from build123d import *

# Parameters (mm, degrees)
SKETCH1_W           = 12
SKETCH1_H           = 12
SKETCH1_W_2         = 3.175
SKETCH1_H_2         = 6
SKETCH1_W_3         = 6
SKETCH1_H_3         = 3.125
BOSS_EXTRUDE1_DEPTH = 1.5875


with BuildPart() as part:
    # Sketch1 → Boss-Extrude1 (new, symmetric)
    with BuildSketch(Plane.XY):
        Polygon((45.675, 0), (45.675, 4.5), (42.5, 4.5), (42.5, 13.5), (45.675, 13.5), (45.675, 22.5), (42.5, 22.5), (42.5, 31.5), (-42.5, 31.5), (-42.5, 22.5), (-45.675, 22.5), (-45.675, 13.5), (-42.5, 13.5), (-42.5, 4.5), (-45.675, 4.5), (-45.675, -4.5), (-42.5, -4.5), (-42.5, -13.5), (-45.675, -13.5), (-45.675, -22.5), (-42.5, -22.5), (-42.5, -31.5), (42.5, -31.5), (42.5, -22.5), (45.675, -22.5), (45.675, -13.5), (42.5, -13.5), (42.5, -4.5), (45.675, -4.5), align=None)
        with Locations((0, -16.5)):
            Rectangle(SKETCH1_W, SKETCH1_H, mode=Mode.SUBTRACT)
        with Locations((0, 16.5)):
            Rectangle(SKETCH1_W, SKETCH1_H, mode=Mode.SUBTRACT)
        with Locations((14.166666667, -21)):
            Rectangle(SKETCH1_W_2, SKETCH1_H_2, mode=Mode.SUBTRACT)
        with Locations((14.166666667, 0)):
            Rectangle(SKETCH1_W_2, SKETCH1_H_2, mode=Mode.SUBTRACT)
        Polygon((31.333333333, 1.5625), (31.333333333, 0), (31.333333333, -1.5625), (25.333333333, -1.5625), (25.333333333, 1.5625), align=None, mode=Mode.SUBTRACT)
        with Locations((14.166666667, 21)):
            Rectangle(SKETCH1_W_2, SKETCH1_H_2, mode=Mode.SUBTRACT)
        with Locations((-14.166666667, 21)):
            Rectangle(SKETCH1_W_2, SKETCH1_H_2, mode=Mode.SUBTRACT)
        with Locations((-14.166666667, -21)):
            Rectangle(SKETCH1_W_2, SKETCH1_H_2, mode=Mode.SUBTRACT)
        with Locations((-28.333333333, 0)):
            Rectangle(SKETCH1_W_3, SKETCH1_H_3, mode=Mode.SUBTRACT)
        with Locations((-14.166666667, 0)):
            Rectangle(SKETCH1_W_2, SKETCH1_H_2, mode=Mode.SUBTRACT)
    extrude(amount=BOSS_EXTRUDE1_DEPTH, both=True)


solid = part.part
Read the model definition and answer for the solid it produces. Units are mm, in the model's axes. A direction names the side the tool comes from. Round coordinates to 2 decimals unless told otherwise and drop trailing zeros. Write each loop counter-clockwise with the first axis right and the second up, starting at its lowest first coordinate (ties: lowest second). Pieces come first, ordered by that corner, then holes.
Q1. Find section A-A on x = 3.5. Determine the outline of the cut face in (y, z).
Values:
outline: (-31.5, -1.59) - (-22.5, -1.59) - (-22.5, 1.59) - (-31.5, 1.59) - close; (-10.5, -1.59) - (10.5, -1.59) - (10.5, 1.59) - (-10.5, 1.59) - close; (22.5, -1.59) - (31.5, -1.59) - (31.5, 1.59) - (22.5, 1.59) - close
Q2. Find section C-C on y = 16.5. Determine the outline of the cut face in (x, z) (1 decimal).
Values:
outline: (-45.7, -1.6) - (-6, -1.6) - (-6, 1.6) - (-45.7, 1.6) - close; (6, -1.6) - (45.7, -1.6) - (45.7, 1.6) - (6, 1.6) - close
Q3. Find section B-B on x = -13.5. Determine the outline of the cut face in (y, z), and give its area (3 significant figures).
Values:
outline: (-31.5, -1.59) - (-24, -1.59) - (-24, 1.59) - (-31.5, 1.59) - close; (-18, -1.59) - (-3, -1.59) - (-3, 1.59) - (-18, 1.59) - close; (3, -1.59) - (18, -1.59) - (18, 1.59) - (3, 1.59) - close; (24, -1.59) - (31.5, -1.59) - (31.5, 1.59) - (24, 1.59) - close
area: 143 mm2
Q4. A tool of negligible diameter and unlimited length cuts with its end or side. For faces 1 (the face through (42.5, -9, 0)), 2 (the face through (-15.754, -21, 0)), 3 (the face through (-42.5, 27, 0)), 4 (the face through (-44, -4.5, 0)), from which of +Z, -Z, +X, -X, +Y, -Y can it reach the whole face along a straight path? Write none if from no direction.
Values:
face 1: +Z, -Z, +X
face 2: +Z, -Z
face 3: +Z, -Z, -X, +Y
face 4: +Z, -Z, -X
Q5. Flat-ended cylindrical pins translate along their axes: P1, Ø1, axis at x = 44, z = 0.5, coming from the +Y side; P2, Ø1, axis at x = -44, z = 0, coming from the -Y side. Find the tip coordinate at first contact, or state that the pin passes through.
Values:
P1: stops at y = 22.5
P2: stops at y = -22.5
Q6. Straight lines are drawn through the part: line 1 (Y direction, x = 4, z = 0); line 2 (X direction, y = 2.5, z = -0.65) (3 decimals); line 3 (X direction, y = 15.5, z = 1.5) (3 decimals). For each, find the intervals that lie inside material, in ascending order.
Values:
line 1: y = -31.5 to -22.5, -10.5 to 10.5, 22.5 to 31.5
line 2: x = -45.675 to -15.754, -12.579 to 12.579, 15.754 to 45.675
line 3: x = -45.675 to -6, 6 to 45.675
Q7. The mould has two halves that part along X. Classify faces 5 (the face through (42.5, 9, 0)), 6 (the face through (-14, 3, 0)), 7 (the face through (-45.675, -18, 0)): released by +X, released by -X, zero draft, split by the parting line, or undercut.
Values:
face 5: released by +X
face 6: undercut
face 7: released by -X
Q8. Find section D-D on x = 30. Determine the outline of the cut face in (y, z), and give its area (3 significant figures).
Values:
outline: (-31.5, -1.59) - (-1.56, -1.59) - (-1.56, 1.59) - (-31.5, 1.59) - close; (1.56, -1.59) - (31.5, -1.59) - (31.5, 1.59) - (1.56, 1.59) - close
area: 190 mm2
